Here's how the part is built. I have some questions about the finished solid (model axes, mm). A direction names the side the tool comes from. Coordinates: 2 decimals unless noted, no trailing zeros. Loops run counter-clockwise (first coordinate to the right, second up) from the corner with the lowest first, then second, coordinate; pieces in that order, holes last. Notation, with made-up numbers: (24, 52.5) -> (45, 52.5) arc R16 ccw to (45, 80.5) -> close; hole circle Ø10 at (-26.75, 71.5). An arc over 180 degrees is marked (long way). Answer as a JSON object with one key per item and string values. Group by question number.
Q1. I want a section at B-B on y = 24. Write out the boundary of the cut face in (x, z), then the cut area to 3 significant figures.
Q2. I'm going to push flat-ended pins straight in: pin 1 (2.5 mm diameter, centred on x = 25.675, y = 25.675, fed in from +Z); pin 2 (3.5 mm diameter, centred on x = 5, y = 3, fed in from +Z); pin 3 (0.6 mm diameter, centred on x = 3.5, z = 2, fed in from -Y). Where does each tip first touch, or does it pass through?
Q3. I want a section at D-D on z = 0.5. Write out the boundary of the cut face in (x, y) (3 decimals), then the cut area to 3 significant figures.
Q4. I want a section at A-A on z = 2. Write out the boundary of the cut face in (x, y) (3 decimals).
Q5. I need wall thicknesses on line 1 (Y direction, x = 10.25, z = 1.25); line 2 (Y direction, x = 3, z = 2); line 3 (Y direction, x = 12.5, z = -1). Which ranges of each line are inside material? Lowest first, please.
Q6. I want a section at C-C on x = 2.5. Write out the boundary of the cut face in (y, z), then the cut area to 3 significant figures.
Q7. Thinking about a two-plate mould opening in Y: for faces 1 (the flat face through (18.55, 25, -3)), 2 (the flat face through (14, 23.55, 2)), 3 (the flat face through (14, 27.85, 1)), which applies, released by +Y, released by -Y, zero draft, split by the parting line, or undercut?
Q8. On a 3-axis mill with a long thin cutter (end or side, diameter ignored), from which of +Z, -Z, +X, -X, +Y, -Y can I reach the whole of each face in a straight line? I mean faces 4 (the flat face through (7.675, 2, 2)), 5 (the flat face through (14, 5, 2.5)), 6 (the flat face through (20.175, 2, 2)). Say none if no direction works.
Autodesk Fusion 360 part; units mm, degrees
sketch "Sketch1" plane through (0, 0, 0) normal (0, 0, 1) x (1, 0, 0)
  line L0 (0, 0) -> (27.85, 0)
  line L1 (27.85, 0) -> (27.85, 27.85)
  line L2 (27.85, 27.85) -> (0, 27.85)
  line L3 (0, 27.85) -> (0, 0)
  dimension "d1" = 27.85
  dimension "d2" = 27.85
extrude "Extrude1" add sketch "Sketch1" along normal blind 1.2
sketch "Sketch2" plane through (0, 0, 1.2) normal (0, 0, 1) x (-1, 0, 0)
  line L0 (0, -27.85) -> (0, 0)
  line L1 (0, 0) -> (-27.85, 0)
  line L2 (-27.85, 0) -> (-27.85, -27.85)
  line L3 (-27.85, -27.85) -> (0, -27.85)
  circle A0 centre (-2.175, -25.675) radius 1
  circle A1 centre (-2.175, -2.175) radius 1
  circle A2 centre (-25.675, -25.675) radius 1
  circle A3 centre (-25.675, -2.175) radius 1
  line L4 (0, -24.675) -> (-27.85, -24.675) construction
  line L5 (0, -3.175) -> (-27.85, -3.175) construction
  line L6 (-24.675, 0) -> (-24.675, -27.85) construction
  line L7 (-3.175, 0) -> (-3.175, -27.85) construction
  line L8 (-24.675, -13.925) -> (-27.85, -13.925) construction
  line L9 (-3.175, -13.925) -> (0, -13.925) construction
  line L10 (-13.925, -24.675) -> (-13.925, -27.85) construction
  line L11 (-13.925, -3.175) -> (-13.925, 0) construction
  dimension "d5" = 2
  dimension "d6" = 21.5
  dimension "d7" = 21.5
extrude "Extrude2" cut sketch "Sketch2" against normal through all contours A0 | A1 | A2 | A3
sketch "Sketch3" plane through (0, 0, 1.2) normal (0, 0, 1) x (-1, 0, 0)
  circle A0 centre (-25.675, -2.175) radius 1
  circle A1 centre (-25.675, -25.675) radius 1
  circle A2 centre (-2.175, -2.175) radius 1
  circle A3 centre (-2.175, -25.675) radius 1
  line L0 (0, -27.85) -> (0, 0)
  line L1 (0, 0) -> (-27.85, 0)
  line L2 (-27.85, 0) -> (-27.85, -27.85)
  line L3 (-27.85, -27.85) -> (0, -27.85)
  line L4 (0, -23.55) -> (-27.85, -23.55)
  line L5 (-27.85, -23.55) -> (-27.85, -4.55)
  line L6 (-27.85, -4.55) -> (0, -4.55)
  line L7 (0, -4.55) -> (0, -23.55)
  line L8 (-7.675, -4.55) -> (-20.175, -4.55)
  line L9 (-20.175, -4.55) -> (-20.175, 0)
  line L10 (-20.175, 0) -> (-7.675, 0)
  line L11 (-7.675, 0) -> (-7.675, -4.55)
  line L12 (-13.925, 0) -> (-13.925, -4.55) construction
  dimension "d9" = 19
  dimension "d10" = 4.3
  dimension "d13" = 12.5
extrude "Extrude3" add sketch "Sketch3" along normal blind 1.5 contours L0 L2 L4 L5 L6 L7 L8
extrude "Extrude4" add sketch "Sketch3" along normal blind 1.3 contours L1 L6 L8 L9 L10 L11
sketch "Sketch4" plane through (0, 0, 1.2) normal (0, 0, 1) x (-1, 0, 0)
  line L0 (0, -23.55) -> (-27.85, -23.55)
  line L1 (-27.85, -23.55) -> (-27.85, -27.85)
  line L2 (-27.85, -27.85) -> (0, -27.85)
  line L3 (0, -27.85) -> (0, -23.55)
  circle A0 centre (-25.675, -25.675) radius 1
  circle A1 centre (-2.175, -25.675) radius 1
  line L4 (-9.3, -27.35) -> (-18.55, -27.35)
  line L5 (-18.55, -27.35) -> (-18.55, -25.85)
  line L6 (-18.55, -25.85) -> (-9.3, -25.85)
  line L7 (-9.3, -25.85) -> (-9.3, -27.35)
  line L8 (-13.925, -27.85) -> (-13.925, -27.35) construction
  dimension "d16" = 2
  dimension "d17" = 1.5
  dimension "d18" = 9.25
extrude "Extrude5" add sketch "Sketch4" along normal blind 1.5 contours L4 L5 L6 L7
extrude "Extrude6" add 1 faces at (15.4667, 26.35, 2.7) along direction (0, 0, -1) blind 7
sketch "Sketch5" plane through (0, 25.85, 0) normal (0, -1, 0) x (1, 0, 0)
  line L0 (18.55, 0) -> (9.3, 0)
  line L1 (9.3, 0) -> (9.3, -4.3)
  line L2 (9.3, -4.3) -> (18.55, -4.3)
  line L3 (18.55, -4.3) -> (18.55, 0)
  line L4 (9.3, -2.8) -> (18.55, -2.8)
  dimension "d23" = 1.5
extrude "Extrude7" add sketch "Sketch5" along normal blind 4 contours L1 L2 L3 L4
sketch "Sketch6" plane through (0, 0, 2.7) normal (0, 0, 1) x (-1, 0, 0)
  line L0 (0, -4.55) -> (-27.85, -4.55)
  line L1 (-27.85, -4.55) -> (-27.85, -23.55)
  line L2 (-27.85, -23.55) -> (0, -23.55)
  line L3 (0, -23.55) -> (0, -4.55)
  line L4 (0, -8.95) -> (-27.85, -8.95)
  dimension "d26" = 14.6
extrude "Extrude8" cut sketch "Sketch6" against normal up to surface (0.2 mm away) contours L0 L1 L3 L4
Result set:
{
 "1": {"outline": "(0, 0) -> (27.85, 0) -> (27.85, 1.2) -> (0, 1.2) -> close; (9.3, -4.3) -> (18.55, -4.3) -> (18.55, -2.8) -> (9.3, -2.8) -> close", "area": "47.3 mm²"},
 "2": {"pin 1": "stops at z = 1.2", "pin 2": "stops at z = 2.5", "pin 3": "stops at y = 4.55"},
 "3": {"outline": "(0, 0) -> (27.85, 0) -> (27.85, 27.85) -> (0, 27.85) -> close; hole circle Ø2 at (2.175, 2.175); hole circle Ø2 at (2.175, 25.675); hole circle Ø2 at (25.675, 2.175); hole circle Ø2 at (25.675, 25.675)", "area": "763 mm²"},
 "4": {"outline": "(0, 4.55) -> (7.675, 4.55) -> (7.675, 0) -> (20.175, 0) -> (20.175, 4.55) -> (27.85, 4.55) -> (27.85, 23.55) -> (0, 23.55) -> close; (9.3, 25.85) -> (18.55, 25.85) -> (18.55, 27.35) -> (9.3, 27.35) -> close"},
 "5": {"line 1": "y = 0 to 23.55, 25.85 to 27.35", "line 2": "y = 4.55 to 23.55", "line 3": "y = 25.85 to 27.35"},
 "6": {"outline": "(0, 0) -> (1.23, 0) -> (1.23, 1.2) -> (0, 1.2) -> close; (3.12, 0) -> (24.73, 0) -> (24.73, 1.2) -> (23.55, 1.2) -> (23.55, 2.7) -> (8.95, 2.7) -> (8.95, 2.5) -> (4.55, 2.5) -> (4.55, 1.2) -> (3.12, 1.2) -> close; (26.62, 0) -> (27.85, 0) -> (27.85, 1.2) -> (26.62, 1.2) -> close", "area": "56.5 mm²"},
 "7": {"face 1": "zero draft", "face 2": "undercut", "face 3": "released by +Y"},
 "8": {"face 4": "+Z, -X, -Y", "face 5": "+Z, +X, -X, -Y", "face 6": "+Z, +X, -Y"}
}
